Here's how the part is built. I have some questions about the finished solid (model axes, mm). A direction names the side the tool comes from. Round coordinates to 2 decimals unless told otherwise and drop trailing zeros. Write each loop counter-clockwise with the first axis right and the second up, starting at its lowest first coordinate (ties: lowest second). Pieces come first, ordered by that corner, then holes. Notation, with made-up numbers: M 76.5,8 L 82.5,8 A18 ccw 82.5,35 Z; hole C 63.25,64 d1. An arc over 180 degrees is marked long. Write item = value, one per line. Start each with the question number.
(1) If we mould it in two halves opening along Z, with no side actions, what happens to faces 1 (the cylindrical face through (1.61, 19.93, 139.2)), 2 (the flat face through (3, 26, 304.8)), 3 (the cylindrical face through (49.23, 19.93, 139.2)), 4 (the flat face through (26, 47.625, 150))? For each: released by +Z, released by -Z, zero draft, split by the parting line, or undercut.
(2) I want a section at A-A (z = 152.4). List the corners of the cut face in (x, y) for me (1 decimal), and give its area (3 significant figures).
(3) I need wall thicknesses on line 1 along X through (y, z) = (22, 32.5) (3 decimals); line 2 along Y through (x, z) = (1, 152). Which ranges of each line are inside material? Lowest first, please.
(4) I want a section at B-B (y = 7.5). List the corners of the cut face in (x, z) for me (3 decimals).
(5) On a 3-axis mill with a long thin cutter (end or side, diameter ignored), from which of +Z, -Z, +X, -X, +Y, -Y can I reach the whole of each face in a straight line? I mean faces 5 (the flat face through (3.175, 41, 150)), 6 (the flat face through (26, 50.8, 150)). Say none if no direction works.
(6) I want a section at D-D (z = 56). List the corners of the cut face in (x, y) for me (3 decimals).
(7) Will this pin go through, and if not, where does the flat tip stop? pin 1 Ø2 at (y, z) = (11.5, 126.5) entering from -X.
Autodesk Inventor part; units mm, degrees
ref_plane "YZ Plane" through (0, 0, 0) normal (1, 0, 0) x (0, 1, 0)
ref_plane "XZ Plane" through (0, 0, 0) normal (0, 1, 0) x (-1, 0, 0)
ref_plane "XY Plane" through (0, 0, 0) normal (0, 0, 1) x (1, 0, 0)
sketch "Sketch1" plane through (0, 0, 0) normal (0, 0, 1) x (1, 0, 0)
  line L0 (0, 0) -> (50.8, 0)
  line L1 (50.8, 0) -> (50.8, 50.8)
  line L2 (50.8, 50.8) -> (0, 50.8)
  line L3 (0, 50.8) -> (0, 0)
  line L4 (3.175, 3.175) -> (47.625, 3.175)
  line L5 (47.625, 3.175) -> (47.625, 47.625)
  line L6 (47.625, 47.625) -> (3.175, 47.625)
  line L7 (3.175, 47.625) -> (3.175, 3.175)
  dimension "d0" = 50.8
  dimension "d1" = 50.8
  dimension "d2" = 44.45
  dimension "d3" = 44.45
  dimension "d4" = 3.175
  dimension "d5" = 3.175
extrude "Extrusion1" add sketch "Sketch1" along normal blind 304.8
sketch "Sketch2" plane through (50.8, 0, 0) normal (1, 0, 0) x (0, 0, -1)
  line L0 (0, 0) -> (0, 50.8)
  line L1 (0, 50.8) -> (-304.8, 50.8)
  circle A0 centre (-152.4, 25.4) radius 14.2875
  dimension "d8" = 28.575
  dimension "d9" = 25.4
  dimension "d10" = 152.4
extrude "Extrusion2" cut sketch "Sketch2" against normal through all
properties part number "Frame Segment"
Returned:
q1.face_1 = undercut
q1.face_2 = released by +Z
q1.face_3 = undercut
q1.face_4 = zero draft
q2.outline = M 0,0 L 50.8,0 L 50.8,11.1 L 47.6,11.1 L 47.6,3.2 L 3.2,3.2 L 3.2,11.1 L 0,11.1 Z; M 0,39.7 L 3.2,39.7 L 3.2,47.6 L 47.6,47.6 L 47.6,39.7 L 50.8,39.7 L 50.8,50.8 L 0,50.8 Z
q2.area = 423 mm²
q3.line_1 = 0 to 3.175, 47.625 to 50.8
q3.line_2 = 0 to 11.12, 39.68 to 50.8
q4.outline = M 0,0 L 3.175,0 L 3.175,304.8 L 0,304.8 Z; M 47.625,0 L 50.8,0 L 50.8,304.8 L 47.625,304.8 Z
q5.face_5 = +Z, -Z
q5.face_6 = +Z, -Z, +X, -X, +Y
q6.outline = M 0,0 L 50.8,0 L 50.8,50.8 L 0,50.8 Z; hole M 3.175,3.175 L 47.625,3.175 L 47.625,47.625 L 3.175,47.625 Z
q7.pin_1 = 0
